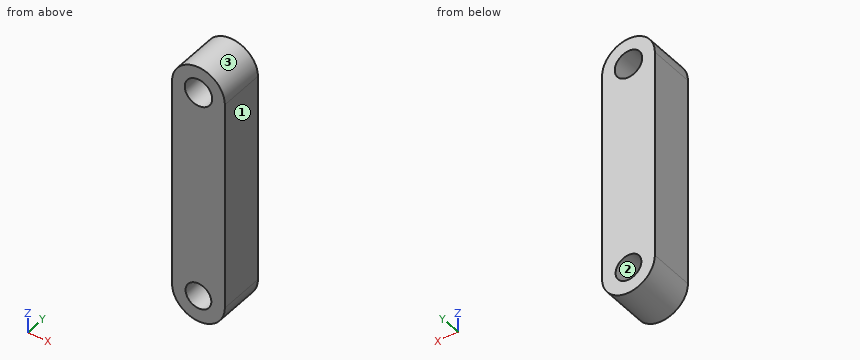
from build123d import *

# Parameters (mm, degrees)
BOSS_EXTRUDE1_DEPTH              = 5.461
M3_CLEARANCE_HOLE_CLEARANCE_D    = 3.3
M3_CLEARANCE_HOLE_INTERFERENCE_D = 3.1


with BuildPart() as part:
    # Sketch1 → Boss-Extrude1 (new body)
    with BuildSketch(Plane(origin=(0, 0, 0), x_dir=(1, 0, 0), z_dir=(0, 1, 0))):
        with BuildLine():
            Line((-3.175, -12.7), (-3.175, 12.7))
            ThreePointArc((-3.175, 12.7), (0, 15.875), (3.175, 12.7))
            Line((3.175, 12.7), (3.175, -12.7))
            ThreePointArc((3.175, -12.7), (0, -15.875), (-3.175, -12.7))
        make_face()
    extrude(amount=BOSS_EXTRUDE1_DEPTH)

    # M3 Clearance Hole clearance (through all)
    with Locations(Plane(origin=(0, 5.461, 0), x_dir=(1, 0, 0), z_dir=(0, 1, 0))):
        with Locations((0, -12.7)):
            Hole(M3_CLEARANCE_HOLE_CLEARANCE_D / 2)

    # M3 Clearance Hole interference (through all)
    with Locations(Plane(origin=(0, 5.461, 0), x_dir=(1, 0, 0), z_dir=(0, 1, 0))):
        with Locations((0, 12.7)):
            Hole(M3_CLEARANCE_HOLE_INTERFERENCE_D / 2)


solid = part.part
Can you work these out from the model? Positions are in its coordinate system, mm. Face numbers are marked on the shaded views. Give positions to 0.01 mm unless a question says otherwise; leave off trailing zeros. Loops run counter-clockwise (first coordinate to the right, second up) from the corner with the lowest first, then second, coordinate; pieces in that order, holes last. Notation, with made-up numbers: (45.25, -8.75) - (96.25, -8.75) arc R26 cw to (96.25, 25.25) - close; hole circle Ø6 at (49.25, 16.25). An arc over 180 degrees is marked (long way). Answer as a JSON object with one key per item and string values.
Q1. Imagine slicing it at B-B on y = 0.7. Write out the boundary of the cut face in (x, z) (3 decimals).
Geometry says:
{"outline": "(-3.175, -12.7) arc R3.175 ccw to (3.175, -12.7) - (3.175, 12.7) arc R3.175 ccw to (-3.175, 12.7) - close; hole circle Ø3.3 at (0, 12.7); hole circle Ø3.1 at (0, -12.7)"}
Q2. Imagine slicing it at C-C on x = -2.25. Write out the boundary of the cut face in (y, z), plus the area to 3 significant figures.
Geometry says:
{"outline": "(0, -14.94) - (5.46, -14.94) - (5.46, 14.94) - (0, 14.94) - close", "area": "163 mm²"}
Q3. If we mould it in two halves opening along X, with no side actions, what happens to the marked faces 1, 2 and 3? For each: pulls with the +X half, pulls with the -X half, needs draft (parallel to the pull), parting line crosses it, or undercut.
Geometry says:
{"face 1": "pulls with the +X half", "face 2": "undercut", "face 3": "parting line crosses it"}
Q4. Will this pin go through, and if not, where does the flat tip stop? P1, Ø2.5, axis at x = 0, z = -12.7, coming from the -Y side.
Geometry says:
{"P1": "through"}
Q5. Imagine slicing it at A-A on x = 0. Write out the boundary of the cut face in (y, z) (3 decimals).
Geometry says:
{"outline": "(0, -15.875) - (5.461, -15.875) - (5.461, -14.25) - (0, -14.25) - close; (0, -11.15) - (5.461, -11.15) - (5.461, 11.05) - (0, 11.05) - close; (0, 14.35) - (5.461, 14.35) - (5.461, 15.875) - (0, 15.875) - close"}
Q6. If I drill on L1, parallel to Z at x = 0, y = 3.3 (3 decimals); L2, parallel to X at y = 2.1, z = 12.7 (3 decimals); L3, parallel to X at y = 1.8, z = -12.7 (3 decimals), over which ranges is the centre line in solid material (lowest first)?
Geometry says:
{"L1": "-15.875 to -14.25, -11.15 to 11.05, 14.35 to 15.875", "L2": "-3.175 to -1.65, 1.65 to 3.175", "L3": "-3.175 to -1.55, 1.55 to 3.175"}
